```python
from build123d import *

# Parameters (mm, degrees)
BOSS_EXTRUDE1_DEPTH = 6
SKETCH2_R           = 1.75
CUT_EXTRUDE1_DEPTH  = 6
SKETCH3_R           = 3.175
CUT_EXTRUDE2_DEPTH  = 3


with BuildPart() as part:
    # Sketch1 → Boss-Extrude1 (new body)
    with BuildSketch(Plane(origin=(0, 0, 0), x_dir=(1, 0, 0), z_dir=(0, 1, 0))):
        Polygon((-75, -45), (75, -45), (75, -22.5), (81, -22.5), (81, -7.5), (75, -7.5), (75, 7.5), (81, 7.5), (81, 22.5), (75, 22.5), (75, 45), (-75, 45), (-75, 22.5), (-81, 22.5), (-81, 7.5), (-75, 7.5), (-75, -7.5), (-81, -7.5), (-81, -22.5), (-75, -22.5), align=None)
    extrude(amount=BOSS_EXTRUDE1_DEPTH)

    # Sketch2 → Cut-Extrude1 (cut)
    with BuildSketch(Plane(origin=(0, 6, 0), x_dir=(1, 0, 0), z_dir=(0, 1, 0))):
        with Locations(Location((32.5, 37.5, 0), (0, 0, 270))):
            Circle(SKETCH2_R)
        with Locations(Location((32.5, -37.5, 0), (0, 0, 270))):
            Circle(SKETCH2_R)
        with Locations(Location((-12.5, 37.5, 0), (0, 0, 270))):
            Circle(SKETCH2_R)
        with Locations(Location((-12.5, -37.5, 0), (0, 0, 270))):
            Circle(SKETCH2_R)
    extrude(amount=-CUT_EXTRUDE1_DEPTH, mode=Mode.SUBTRACT)

    # Sketch3 → Cut-Extrude2 (cut)
    with BuildSketch(Plane(origin=(0, 6, 0), x_dir=(1, 0, 0), z_dir=(0, 1, 0))):
        with Locations(Location((-12.5, 37.5, 0), (0, 0, 270))):
            Circle(SKETCH3_R)
        with Locations(Location((32.5, 37.5, 0), (0, 0, 270))):
            Circle(SKETCH3_R)
        with Locations(Location((32.5, -37.5, 0), (0, 0, 270))):
            Circle(SKETCH3_R)
        with Locations(Location((-12.5, -37.5, 0), (0, 0, 270))):
            Circle(SKETCH3_R)
    extrude(amount=-CUT_EXTRUDE2_DEPTH, mode=Mode.SUBTRACT)


solid = part.part
```
Geometry: final body of the model. Coordinates: model frame, mm. A direction names the side the tool comes from. Round coordinates to 2 decimals unless told otherwise and drop trailing zeros. Write each loop counter-clockwise with the first axis right and the second up, starting at its lowest first coordinate (ties: lowest second). Pieces come first, ordered by that corner, then holes. Notation, with made-up numbers: M 86,17 L 125,17 A21 cw 125,49 Z; hole C 23.25,16 d9. An arc over 180 degrees is marked long. Answer in a Markdown table with one row per item. Add a question column.
(1) Contact query for flat-ended pins moving along their axis: pin 1 (3 mm diameter, centred on y = 3, z = 31.5, fed in from +X); pin 2 (3 mm diameter, centred on x = 32.5, z = 37.5, fed in from +Y); pin 3 (1.9 mm diameter, centred on x = -14, z = -39, fed in from +Y); pin 4 (1.8 mm diameter, centred on x = 77, y = 3.5, fed in from +Z). Output: stop coordinate, or through.
(2) Cut plane D-D, the plane z = 2. Return the cut outline in (x, y).
(3) Reachability of faces 1 (the face through (78, 3, -7.5)), 2 (the face through (-78, 3, 7.5)), 3 (the face through (-13.72, 4.52, -34.57)), 4 (the face through (-75, 3, 34)) from +Z, -Z, +X, -X, +Y, -Y: full face, straight path, thin tool, end or side. Return the list, or none.
(4) Ray query, L1, parallel to X at y = 4.4, z = -37.5 (3 decimals); L2, parallel to X at y = 2.25, z = -37.5; L3, parallel to X at y = 4.65, z = 23. Return the intervals inside material, ascending.
(5) Cut plane C-C, the plane x = -12.5. Return the cut outline in (y, z) (3 decimals), then the cut area to 3 significant figures.
(6) Cut plane A-A, the plane y = 4.05. Return the cut outline in (x, z) (3 decimals).
(7) Cut plane B-B, the plane z = -37.5. Return the cut outline in (x, y) (3 decimals).
Established:
| question | item | result |
|---|---|---|
| 1 | pin 1 | x = 75 |
| 1 | pin 2 | through |
| 1 | pin 3 | y = 3 |
| 1 | pin 4 | z = 22.5 |
| 2 | outline | M -75,0 L 75,0 L 75,6 L -75,6 Z |
| 3 | face 1 | +X, +Y, -Y |
| 3 | face 2 | -X, +Y, -Y |
| 3 | face 3 | +Y |
| 3 | face 4 | +Z, -X, +Y, -Y |
| 4 | L1 | -75 to -15.675, -9.325 to 29.325, 35.675 to 75 |
| 4 | L2 | -75 to -14.25, -10.75 to 30.75, 34.25 to 75 |
| 4 | L3 | -75 to 75 |
| 5 | outline | M 0,-45 L 6,-45 L 6,-40.675 L 3,-40.675 L 3,-39.25 L 0,-39.25 Z; M 0,-35.75 L 3,-35.75 L 3,-34.325 L 6,-34.325 L 6,34.325 L 3,34.325 L 3,35.75 L 0,35.75 Z; M 0,39.25 L 3,39.25 L 3,40.675 L 6,40.675 L 6,45 L 0,45 Z |
| 5 | area | 481 mm² |
| 6 | outline | M -81,-22.5 L -75,-22.5 L -75,-45 L 75,-45 L 75,-22.5 L 81,-22.5 L 81,-7.5 L 75,-7.5 L 75,7.5 L 81,7.5 L 81,22.5 L 75,22.5 L 75,45 L -75,45 L -75,22.5 L -81,22.5 L -81,7.5 L -75,7.5 L -75,-7.5 L -81,-7.5 Z; hole C -12.5,-37.5 d6.35; hole C -12.5,37.5 d6.35; hole C 32.5,-37.5 d6.35; hole C 32.5,37.5 d6.35 |
| 7 | outline | M -75,0 L -14.25,0 L -14.25,3 L -15.675,3 L -15.675,6 L -75,6 Z; M -10.75,0 L 30.75,0 L 30.75,3 L 29.325,3 L 29.325,6 L -9.325,6 L -9.325,3 L -10.75,3 Z; M 34.25,0 L 75,0 L 75,6 L 35.675,6 L 35.675,3 L 34.25,3 Z |
